Geometry check sheet. Reference: the model listing, model coordinates, mm. Round coordinates to 2 decimals unless told otherwise and drop trailing zeros. Write each loop counter-clockwise with the first axis right and the second up, starting at its lowest first coordinate (ties: lowest second). Pieces come first, ordered by that corner, then holes. Notation, with made-up numbers: (82.25, 8) - (88.25, 8) arc R22 cw to (88.25, 26) - close; hole circle Ø8 at (50, -30). An arc over 180 degrees is marked (long way). Return JSON: item names as keys, results as strings.
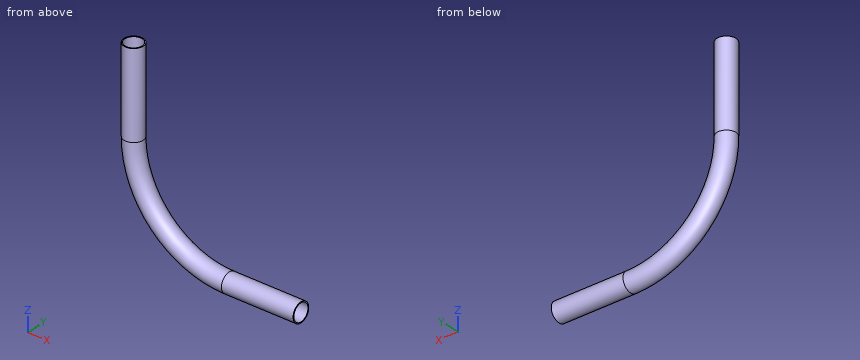
```python
from build123d import *

# Parameters (mm, degrees)
F2_R   = 20
F2_R_2 = 18


with BuildPart() as f3:
    # F3: sweep along a path in F0
    with BuildLine(Plane.XZ) as f3_path:
        Line((0, 377), (0, 200))
        ThreePointArc((0, 200), (58.578644, 58.578644), (200, 0))
        Line((200, 0), (350, 0))
    # F2 (on plane+point) → F3 (sweep)
    with BuildSketch(Plane.XY.offset(377)):
        Circle(F2_R)
        Circle(F2_R_2, mode=Mode.SUBTRACT)
    sweep(path=f3_path.line)


solid = f3.part
```
(1) Section check A-A, the plane z = 256. Enter the section's corners in (x, y).
Response values:
{"outline": "circle Ø40 at (0, 0); hole circle Ø36 at (0, 0)"}
(2) Gauge pin test, flat ends, axial feed: pin 1 (2 mm diameter, centred on x = 166, y = -0.5, fed in from +Z); pin 2 (1.5 mm diameter, centred on x = 270.5, y = 14.5, fed in from +Z); pin 3 (21.5 mm diameter, centred on x = 0, y = 0, fed in from -Z). Record the tip position at first contact, or that the pin passes through.
Response values:
{"pin 1": "stops at z = 23.43", "pin 2": "stops at z = 14.52", "pin 3": "stops at z = 87.82"}
(3) Material ranges on line 1 along Y through (x, z) = (0, 235.5); line 2 along Z through (x, y) = (311, 12), recorded low to high. Write a range as [from, to].
Response values:
{"line 1": "y = [-20, -18], [18, 20]", "line 2": "z = [-16, -13.42], [13.42, 16]"}
